Geometry check sheet. Reference: the model listing, model coordinates, mm. A direction names the side the tool comes from. Coordinates: 2 decimals unless noted, no trailing zeros. Write each loop counter-clockwise with the first axis right and the second up, starting at its lowest first coordinate (ties: lowest second). Pieces come first, ordered by that corner, then holes. Notation, with made-up numbers: (61, -28) -> (67, -28) arc R14 cw to (67, -6) -> close; hole circle Ø1 at (-7, 7.25). An arc over 180 degrees is marked (long way). One line per question, with ' | ' between items.
```python
from build123d import *

# Parameters (mm, degrees)
P_IDAT_VYSUNUT_M1_DEPTH  = 85.5
SKICA2_W                 = 49
SKICA2_H                 = 35
SKICA2_W_2               = 60
ODEBRAT_VYSUNUT_M1_DEPTH = 144.057680675
SKICA3_W                 = 5
SKICA3_H                 = 49
SKICA3_H_2               = 60
ODEBRAT_VYSUNUT_M2_DEPTH = 22
SKICA4_W                 = 94.5
SKICA4_H                 = 131
ODEBRAT_VYSUNUT_M3_DEPTH = 160.73897458
ZAOBLIT1_R               = 5
ZAOBLIT2_R               = 20
ZAOBLIT3_R               = 5
P_IDAT_VYSUNUT_M2_DEPTH  = 3
SKICA6_W                 = 12.8
SKICA6_H                 = 3
P_IDAT_VYSUNUT_M3_DEPTH  = 20
ZAOBLIT4_R               = 5


with BuildPart() as part:
    # Skica1 → Přidat vysunutím1 (new, symmetric)
    with BuildSketch(Plane.XY):
        Polygon((-27.8, 65), (-27.8, 8), (-122.3, 8), (-122.3, 0), (0, 0), (0, 8), (-5, 8), (-5, 65), (-10, 65), (-10, 30), (-22.8, 30), (-22.8, 65), align=None)
    extrude(amount=P_IDAT_VYSUNUT_M1_DEPTH, both=True)

    # Skica2 → Odebrat vysunutím1 (cut, through all)
    with BuildSketch(Plane.ZY.offset(27.8)):
        with Locations((-61, 47.5)):
            Rectangle(SKICA2_W, SKICA2_H)
        with Locations((55.5, 47.5)):
            Rectangle(SKICA2_W_2, SKICA2_H)
    extrude(amount=-ODEBRAT_VYSUNUT_M1_DEPTH, mode=Mode.SUBTRACT)

    # Skica3 → Odebrat vysunutím2 (cut)
    with BuildSketch(Plane(origin=(0, 30, 0), x_dir=(1, 0, 0), z_dir=(0, 1, 0))):
        with Locations((-25.3, 61)):
            Rectangle(SKICA3_W, SKICA3_H)
        with Locations((-7.5, 61)):
            Rectangle(SKICA3_W, SKICA3_H)
        with Locations((-25.3, -55.5)):
            Rectangle(SKICA3_W, SKICA3_H_2)
        with Locations((-7.5, -55.5)):
            Rectangle(SKICA3_W, SKICA3_H_2)
    extrude(amount=-ODEBRAT_VYSUNUT_M2_DEPTH, mode=Mode.SUBTRACT)

    # Skica4 → Odebrat vysunutím3 (cut, through all)
    with BuildSketch(Plane(origin=(0, 8, 0), x_dir=(1, 0, 0), z_dir=(0, 1, 0))):
        with Locations((-75.05, 0)):
            Rectangle(SKICA4_W, SKICA4_H)
    extrude(amount=-ODEBRAT_VYSUNUT_M3_DEPTH, mode=Mode.SUBTRACT)

    # Zaoblit1
    zaoblit1_edges = [part.edges().sort_by_distance(p)[0] for p in [
        (0, 4, -85.5),
        (-122.3, 4, 65.5),
        (-122.3, 4, -65.5),
        (-122.3, 4, -85.5),
        (-122.3, 4, 85.5),
        (0, 4, 85.5),
    ]]
    fillet(zaoblit1_edges, radius=ZAOBLIT1_R)

    # Zaoblit2
    zaoblit2_edges = [part.edges().sort_by_distance(p)[0] for p in [
        (-27.8, 4, -65.5),
        (-27.8, 4, 65.5),
    ]]
    fillet(zaoblit2_edges, radius=ZAOBLIT2_R)

    # Zaoblit3
    zaoblit3_edges = [part.edges().sort_by_distance(p)[0] for p in [
        (-7.5, 65, -36.5),
        (-25.3, 65, -36.5),
        (-25.3, 65, 25.5),
        (-7.5, 65, 25.5),
    ]]
    fillet(zaoblit3_edges, radius=ZAOBLIT3_R)

    # Skica5 → Přidat vysunutím2 (add)
    with BuildSketch(Plane(origin=(0, 0, -85.5), x_dir=(-1, 0, 0), z_dir=(0, 0, -1))):
        Polygon((22.8, 30), (22.8, 8), (117.3, 8), align=None)
    p_idat_vysunut_m2 = extrude(amount=-P_IDAT_VYSUNUT_M2_DEPTH)

    # Zrcadlit1: Přidat vysunutím2 across plane
    add(p_idat_vysunut_m2.mirror(Plane.XY))

    # Skica6 → Přidat vysunutím3 (add)
    with BuildSketch(Plane(origin=(0, 30, 0), x_dir=(1, 0, 0), z_dir=(0, 1, 0))):
        with Locations((-16.4, 84)):
            Rectangle(SKICA6_W, SKICA6_H)
        with Locations((-16.4, -84)):
            Rectangle(SKICA6_W, SKICA6_H)
    extrude(amount=P_IDAT_VYSUNUT_M3_DEPTH)

    # Zaoblit4
    # the kernel refuses this fillet: 5 mm, written as the material it adds along each edge
    with BuildSketch(Plane(origin=(-22.8, 30, 85.5), x_dir=(0, 1, 0), z_dir=(0, 0, -1)), Plane(origin=(-22.8, 30, -85.5), x_dir=(-0.9739551200282253, -0.22674087450392655, 0), z_dir=(0, 0, 1))) as zaoblit4_piece_1:
        with BuildLine():
            CenterArc((ZAOBLIT4_R * 0.793937122558, -ZAOBLIT4_R), ZAOBLIT4_R, 90, 76.89473101)
            Line((-ZAOBLIT4_R * 0.18001799747, -ZAOBLIT4_R * 0.773259125496), (0, 0))
            Line((0, 0), (ZAOBLIT4_R * 0.793937122558, 0))
        make_face()
    extrude(amount=3)
    # the kernel refuses this fillet: 5 mm, written as the material it takes off along each edge
    with BuildSketch(Plane(origin=(-22.8, 50, -98), x_dir=(1, 0, 0), z_dir=(0, 0, 1)), Plane(origin=(-10, 50, 70), x_dir=(0, -1, 0), z_dir=(0, 0, 1))) as zaoblit4_2_piece_1:
        with BuildLine():
            CenterArc((ZAOBLIT4_R, -ZAOBLIT4_R), ZAOBLIT4_R, 90, 90)
            Line((0, -ZAOBLIT4_R), (0, 0))
            Line((0, 0), (ZAOBLIT4_R, 0))
        make_face()
    extrude(amount=28, mode=Mode.SUBTRACT)
    with BuildSketch(Plane(origin=(-10, 50, -70), x_dir=(0, -1, 0), z_dir=(0, 0, -1)), Plane(origin=(-22.8, 50, 98), x_dir=(1, 0, 0), z_dir=(0, 0, -1))) as zaoblit4_2_piece_2:
        with BuildLine():
            CenterArc((ZAOBLIT4_R, ZAOBLIT4_R), ZAOBLIT4_R, 180, 90)
            Line((0, ZAOBLIT4_R), (0, 0))
            Line((0, 0), (ZAOBLIT4_R, 0))
        make_face()
    extrude(amount=28, mode=Mode.SUBTRACT)


solid = part.part
```
(1) Cross-section at C-C (z = 18.5). Record the cut outline in (x, y).
Answers below:
outline: (-27.8, 0) -> (0, 0) -> (0, 8) -> (-5, 8) -> (-5, 65) -> (-10, 65) -> (-10, 30) -> (-22.8, 30) -> (-22.8, 65) -> (-27.8, 65) -> close
(2) Cross-section at B-B (y = 54). Record the cut outline in (x, z).
Answers below:
outline: (-27.8, -36.5) -> (-22.8, -36.5) -> (-22.8, 25.5) -> (-27.8, 25.5) -> close; (-10, -36.5) -> (-5, -36.5) -> (-5, 25.5) -> (-10, 25.5) -> close
(3) Material ranges on line 1 (X direction, y = 52, z = -27); line 2 (Z direction, x = -61, y = 6); line 3 (X direction, y = 22.5, z = -66), recorded low to high.
Answers below:
line 1: x = -27.8 to -22.8, -10 to -5 | line 2: z = -85.5 to -65.5, 65.5 to 85.5 | line 3: x = -22.8 to -10
(4) Draft check along Z on faces 6 (the face through (-25, 65, -5)), 7 (the face through (-8, 34, -36.5)), 8 (the face through (-33.814, 3.944, -59.797)). Enter one of: pulls with the +Z half, pulls with the -Z half, needs draft (parallel to the pull), parting line crosses it, or undercut.
Answers below:
face 6: needs draft | face 7: pulls with the -Z half | face 8: undercut
(5) Cross-section at A-A (y = 41). Record the cut outline in (x, z), plus the area to 3 significant figures.
Answers below:
outline: (-27.8, -36.5) -> (-22.8, -36.5) -> (-22.8, 25.5) -> (-27.8, 25.5) -> close; (-22.8, -85.5) -> (-10, -85.5) -> (-10, -82.5) -> (-22.8, -82.5) -> close; (-22.8, 82.5) -> (-10, 82.5) -> (-10, 85.5) -> (-22.8, 85.5) -> close; (-10, -36.5) -> (-5, -36.5) -> (-5, 25.5) -> (-10, 25.5) -> close | area: 697 mm²
(6) Cross-section at D-D (x = -46). Record the cut outline in (y, z).
Answers below:
outline: (0, -85.5) -> (24.6, -85.5) -> (24.6, -82.5) -> (8, -82.5) -> (8, -65.42) -> (0, -65.42) -> close; (0, 65.42) -> (8, 65.42) -> (8, 82.5) -> (24.6, 82.5) -> (24.6, 85.5) -> (0, 85.5) -> close
(7) Tool access check on faces 1 (the face through (-72, 8, -72)), 2 (the face through (-10, 19, 56)), 3 (the face through (-23.913, 30.824, -84.021)), 4 (the face through (-27.8, 33, 1)), 5 (the face through (-23.855, 30.898, 84.021)). Record the directions out of +Z, -Z, +X, -X, +Y, -Y that give a thin tool (end or side, any length) a straight path to the whole face; none if there is none.
Answers below:
face 1: -X, +Y | face 2: +Z, +X, +Y | face 3: -Z, -X, +Y | face 4: -X, +Y, -Y | face 5: +Z, -X, +Y
(8) Depth check by flat-ended pin: P1, Ø1.5, axis at y = 40, z = -84.5, coming from the -X side; P2, Ø2.5, axis at x = -26, y = 40, coming from the -Z side; P3, Ø1, axis at y = 52.5, z = -9.5, coming from the -X side. Enter the tip coordinate at first touch or a pass-through.
Answers below:
P1: stops at x = -22.8 | P2: stops at z = -36.5 | P3: stops at x = -27.8
